Verification items for the finished model (mm, model axes). Face numbers are marked on the shaded views. A direction names the side the tool comes from. Give positions to 0.01 mm unless a question says otherwise; leave off trailing zeros. Order: outer loops, then holes, each group sorted by start corner. A loop starts at its lowest first (then second) coordinate and runs counter-clockwise, first axis right, second up. Notation, with made-up numbers: (45, 33) -> (77, 33) arc R18 ccw to (77, 67) -> close; hole circle Ø11 at (-16.75, -9). An arc over 180 degrees is marked (long way). One line per question, with ' | ' between items. Start each with the question number.
Q1. Access from +Z, -Z, +X, -X, +Y, -Y to the whole of each face (thin tool, end or side, straight path). Record for the marked faces 1 and 2.
Q2. Section check A-A on z = -17.75. Record the cut outline in (x, y).
Q3. Material ranges on probe 1 along Z at (x, y) = (-1.65, -0.35); probe 2 along X at (y, z) = (0.05, -14.75); probe 3 along Z at (x, y) = (-0.9, -0.95), recorded low to high. Write a range as [from, to].
Q4. Go/stop test with flat-tipped pins: pin 1 (3 mm diameter, centred on y = -1, z = -19, fed in from -X); pin 2 (3 mm diameter, centred on x = -1.5, z = -18.5, fed in from +Y); pin 3 (0.5 mm diameter, centred on x = -0.5, z = 1, fed in from -Y). Record where each tip stops, or that it passes through.
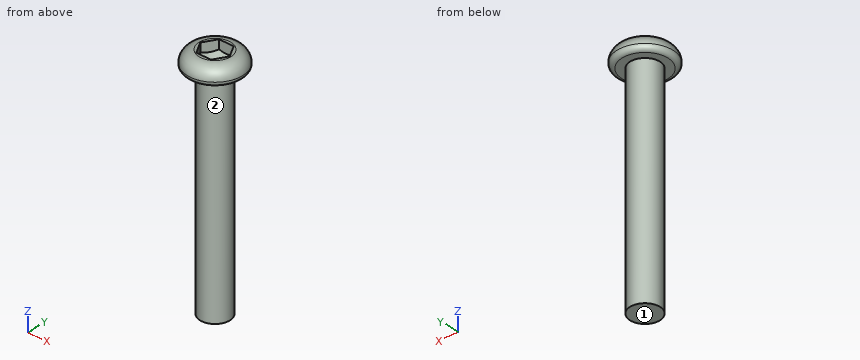
Autodesk Inventor part; units mm, degrees
ref_plane "YZ Plane" through (0, 0, 0) normal (1, 0, 0) x (0, 1, 0)
ref_plane "XZ Plane" through (0, 0, 0) normal (0, 1, 0) x (-1, 0, 0)
ref_plane "XY Plane" through (0, 0, 0) normal (0, 0, 1) x (1, 0, 0)
sketch "Sketch1" plane through (0, 0, 0) normal (0, 0, 1) x (1, 0, 0)
  circle A0 centre (0, 0) radius 2.8
  dimension "d0" = 5.6
extrude "Extrusion1" add sketch "Sketch1" along normal blind 1.7
fillet "Fillet3" radius 0.5 1 edges at (-2.8, 0, 0)
fillet "Fillet4" radius 1.2 1 edges at (-2.8, 0, 1.7)
sketch "Sketch2" plane through (0, 0, 1.7) normal (0, 0, 1) x (1, 0, 0)
  line L0 (-0.75, -1.299) -> (0.75, -1.299)
  line L1 (0.75, -1.299) -> (1.5, 0)
  line L2 (1.5, 0) -> (0.75, 1.299)
  line L3 (0.75, 1.299) -> (-0.75, 1.299)
  line L4 (-0.75, 1.299) -> (-1.5, 0)
  line L5 (-1.5, 0) -> (-0.75, -1.299)
  dimension "d7" = 3
extrude "Extrusion2" cut sketch "Sketch2" against normal blind 1.7
sketch "Sketch3" plane through (0, 0, 0) normal (0, 1, 0) x (-1, 0, 0)
  line L0 (0, 0) -> (1.5, 0)
  line L1 (2.3, 0) -> (-2.3, 0)
  line L2 (1.5, 0) -> (1.5, 0.8)
  line L3 (1.5, 0.8) -> (0, 0)
  line L4 (0, 0) -> (0, 2.432)
  dimension "d13" = 0
  dimension "d14" = 1.5
  dimension "d15" = 0.8
revolve "Revolution2" add sketch "Sketch3" angle 360 about axis through (0, 0, 0) along (0, 0, 1)
sketch "Sketch4" plane through (0, 0, 0) normal (0, 0, -1) x (-1, 0, 0)
  circle A0 centre (0, 0) radius 2.3
  circle A1 centre (0, 0) radius 1.5
  dimension "d18" = 3
extrude "Extrusion3" add sketch "Sketch4" along normal blind 22 contours A1
thread "Thread1"
properties part number "screw_M3_16_hex"
Filled in:
1) face 1: -Z, +X, -X, +Y, -Y | face 2: -Z
2) outline: circle Ø3 at (0, 0)
3) probe 1: [0, 1.7] | probe 2: [-1.5, 1.5] | probe 3: [-22, 0.7]
4) pin 1: x = -1.5 | pin 2: y = 1.5 | pin 3: y = -2.74
